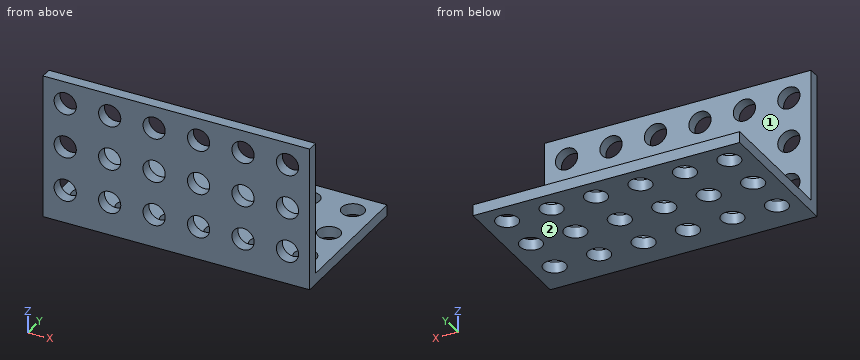
```python
from build123d import *

# Parameters (mm, degrees)
EXTRUDE_1_DEPTH     = 48
SKETCH_2_R          = 2
CUT_EXTRUDE_1_DEPTH = 48
SKETCH_3_R          = 2
CUT_EXTRUDE_3_DEPTH = 48


with BuildPart() as part:
    # 草图1 → 凸台-拉伸1 (new body)
    with BuildSketch(Plane(origin=(0, 0, 0), x_dir=(0, 0, -1), z_dir=(1, 0, 0))):
        Polygon((0, 0), (-26, 0), (-26, 2), (-2, 2), (-2, 26), (0, 26), align=None)
    extrude(amount=EXTRUDE_1_DEPTH)

    # 草图2 → 切除-拉伸1 (cut)
    with BuildSketch(Plane.XY.offset(2)):
        with Locations((4, 22)):
            Circle(SKETCH_2_R)
        with Locations((4, 14)):
            Circle(SKETCH_2_R)
        with Locations((4, 6)):
            Circle(SKETCH_2_R)
        with Locations((12, 22)):
            Circle(SKETCH_2_R)
        with Locations((12, 14)):
            Circle(SKETCH_2_R)
        with Locations((12, 6)):
            Circle(SKETCH_2_R)
        with Locations((20, 22)):
            Circle(SKETCH_2_R)
        with Locations((20, 14)):
            Circle(SKETCH_2_R)
        with Locations((20, 6)):
            Circle(SKETCH_2_R)
        with Locations((28, 22)):
            Circle(SKETCH_2_R)
        with Locations((28, 14)):
            Circle(SKETCH_2_R)
        with Locations((28, 6)):
            Circle(SKETCH_2_R)
        with Locations((36, 22)):
            Circle(SKETCH_2_R)
        with Locations((36, 14)):
            Circle(SKETCH_2_R)
        with Locations((36, 6)):
            Circle(SKETCH_2_R)
        with Locations((44, 22)):
            Circle(SKETCH_2_R)
        with Locations((44, 14)):
            Circle(SKETCH_2_R)
        with Locations((44, 6)):
            Circle(SKETCH_2_R)
    extrude(amount=-CUT_EXTRUDE_1_DEPTH, mode=Mode.SUBTRACT)

    # 草图3 → 切除-拉伸3 (cut)
    with BuildSketch(Plane(origin=(0, 2, 0), x_dir=(1, 0, 0), z_dir=(0, 1, 0))):
        with Locations(Location((4, -22, 0), (0, 0, 270))):
            Circle(SKETCH_3_R)
        with Locations(Location((4, -14, 0), (0, 0, 270))):
            Circle(SKETCH_3_R)
        with Locations(Location((4, -6, 0), (0, 0, 270))):
            Circle(SKETCH_3_R)
        with Locations(Location((12, -6, 0), (0, 0, 270))):
            Circle(SKETCH_3_R)
        with Locations(Location((12, -14, 0), (0, 0, 270))):
            Circle(SKETCH_3_R)
        with Locations(Location((12, -22, 0), (0, 0, 270))):
            Circle(SKETCH_3_R)
        with Locations(Location((20, -6, 0), (0, 0, 270))):
            Circle(SKETCH_3_R)
        with Locations(Location((20, -14, 0), (0, 0, 270))):
            Circle(SKETCH_3_R)
        with Locations(Location((20, -22, 0), (0, 0, 270))):
            Circle(SKETCH_3_R)
        with Locations(Location((28, -6, 0), (0, 0, 270))):
            Circle(SKETCH_3_R)
        with Locations(Location((28, -14, 0), (0, 0, 270))):
            Circle(SKETCH_3_R)
        with Locations(Location((28, -22, 0), (0, 0, 270))):
            Circle(SKETCH_3_R)
        with Locations(Location((36, -6, 0), (0, 0, 270))):
            Circle(SKETCH_3_R)
        with Locations(Location((36, -14, 0), (0, 0, 270))):
            Circle(SKETCH_3_R)
        with Locations(Location((36, -22, 0), (0, 0, 270))):
            Circle(SKETCH_3_R)
        with Locations(Location((44, -6, 0), (0, 0, 270))):
            Circle(SKETCH_3_R)
        with Locations(Location((44, -14, 0), (0, 0, 270))):
            Circle(SKETCH_3_R)
        with Locations(Location((44, -22, 0), (0, 0, 270))):
            Circle(SKETCH_3_R)
    extrude(amount=-CUT_EXTRUDE_3_DEPTH, mode=Mode.SUBTRACT)


solid = part.part
```
Check sheet for the modelled part. Datum: model origin and axes. Units: mm. Face numbers are marked on the shaded views. A direction names the side the tool comes from. Round coordinates to 2 decimals unless told otherwise and drop trailing zeros. Loops run counter-clockwise (first coordinate to the right, second up) from the corner with the lowest first, then second, coordinate; pieces in that order, holes last. Notation, with made-up numbers: M -24,59 L 26,59 A17 cw 26,79 Z; hole C -39.5,-30.75 d5. An arc over 180 degrees is marked long. Answer as a JSON object with one key per item and string values.
1. Gauge pin test, flat ends, axial feed: P1, Ø4.5, axis at x = 44, y = 6, coming from the +Z side; P2, Ø1.5, axis at x = 8, z = 20.5, coming from the +Y side. Record the tip position at first contact, or that the pin passes through.
Reply:
{"P1": "stops at z = 2", "P2": "stops at y = 2"}
2. Section check D-D (x = 32). Record the boundary of the cut face in (y, z).
Reply:
{"outline": "M 0,0 L 26,0 L 26,2 L 2,2 L 2,26 L 0,26 Z"}
3. Access from +Z, -Z, +X, -X, +Y, -Y to the whole of each face (thin tool, end or side, straight path). Record for the marked faces 1 and 2.
Reply:
{"face 1": "+Z, +X, -X, +Y", "face 2": "-Z, +X, -X, +Y, -Y"}
4. Section check A-A (y = 14). Record the boundary of the cut face in (x, z).
Reply:
{"outline": "M 0,0 L 2,0 L 2,2 L 0,2 Z; M 6,0 L 10,0 L 10,2 L 6,2 Z; M 14,0 L 18,0 L 18,2 L 14,2 Z; M 22,0 L 26,0 L 26,2 L 22,2 Z; M 30,0 L 34,0 L 34,2 L 30,2 Z; M 38,0 L 42,0 L 42,2 L 38,2 Z; M 46,0 L 48,0 L 48,2 L 46,2 Z"}
5. Scan lines: line 1 (Y direction, x = 44, z = 1.2); line 2 (Z direction, x = 27.5, y = 1.5); line 3 (Y direction, x = 22, z = 24.75). Record each from-to range of solid material in increasing order.
Reply:
{"line 1": "y = 0 to 4, 8 to 12, 16 to 20, 24 to 26", "line 2": "z = 0 to 4.06, 7.94 to 12.06, 15.94 to 20.06, 23.94 to 26", "line 3": "y = 0 to 2"}
6. Section check C-C (x = 12). State how many separate pieces and enclosed holes the cut face has, plus the area to 3 significant figures.
Reply:
{"separate pieces": "7", "enclosed holes": "0", "area": "52.0 mm²"}
